The listing builds one solid part. Answer for the finished solid, in the listing's coordinates (mm). A direction names the side the tool comes from. Give positions to 0.01 mm unless a question says otherwise; leave off trailing zeros. Order: outer loops, then holes, each group sorted by start corner. A loop starts at its lowest first (then second) coordinate and runs counter-clockwise, first axis right, second up. Notation, with made-up numbers: (-21, 12.5) - (24, 12.5) arc R28 ccw to (24, 38.5) - close; hole circle Ø1 at (8.5, 36). An arc over 180 degrees is marked (long way). Answer in a Markdown table with one row per item.
from build123d import *

# Parameters (mm, degrees)
SKETCH1_R               = 26.19375
BOSS_EXTRUDE1_DEPTH     = 8.397875
SKETCH2_R               = 12.7
BOSS_EXTRUDE2_DEPTH     = 15.08125
BOSS_EXTRUDE3_START     = 6.35
SKETCH3_R               = 26.19375
BOSS_EXTRUDE3_DEPTH     = 6.35
F_1_4_20_TAPPED_HOLE1_D = 5.1054
SKETCH6_W               = 66.50359939
SKETCH6_H               = 67.616646228
CUT_EXTRUDE2_DEPTH      = 7.9375


with BuildPart() as part:
    # Sketch1 → Boss-Extrude1 (new body)
    with BuildSketch(Plane(origin=(0, 0, 0), x_dir=(1, 0, 0), z_dir=(0, 1, 0))):
        with Locations(Location((0, 0, 0), (0, 0, 270))):
            Circle(SKETCH1_R)
    extrude(amount=-BOSS_EXTRUDE1_DEPTH)

    # Sketch2 → Boss-Extrude2 (add)
    with BuildSketch(Plane.XZ.offset(8.397875)):
        with Locations(Location((0, 0, 0), (0, 0, 90))):
            Circle(SKETCH2_R)
    extrude(amount=BOSS_EXTRUDE2_DEPTH)

    # Sketch3 → Boss-Extrude3 (add)
    with BuildSketch(Plane(origin=(0, 0, 0), x_dir=(1, 0, 0), z_dir=(0, 1, 0)).offset(BOSS_EXTRUDE3_START)):
        with Locations(Location((0, 0, 0), (0, 0, 270))):
            Circle(SKETCH3_R)
        with BuildLine():
            ThreePointArc((2.553003524, 16.40046245), (5.651302793, 17.39292157), (7.574526721, 14.768870658))
            ThreePointArc((7.574526721, 14.768870658), (7.926495509, 13.34211974), (8.883198518, 12.226673836))
            ThreePointArc((8.883198518, 12.226673836), (10.239688102, 11.661486946), (11.705373197, 11.767635017))
            ThreePointArc((11.705373197, 11.767635017), (14.795302793, 10.749416694), (14.808845207, 7.496072251))
            ThreePointArc((14.808845207, 7.496072251), (14.25497079, 6.134924448), (14.373317131, 4.670173836))
            ThreePointArc((14.373317131, 4.670173836), (15.138531738, 3.415603465), (16.386688159, 2.639970974))
            ThreePointArc((16.386688159, 2.639970974), (18.288, 0), (16.386688159, -2.639970974))
            ThreePointArc((16.386688159, -2.639970974), (15.138531738, -3.415603465), (14.373317131, -4.670173836))
            ThreePointArc((14.373317131, -4.670173836), (14.25497079, -6.134924448), (14.808845207, -7.496072251))
            ThreePointArc((14.808845207, -7.496072251), (14.795302793, -10.749416694), (11.705373197, -11.767635017))
            ThreePointArc((11.705373197, -11.767635017), (10.239688102, -11.661486946), (8.883198518, -12.226673836))
            ThreePointArc((8.883198518, -12.226673836), (7.926495509, -13.34211974), (7.574526721, -14.768870658))
            ThreePointArc((7.574526721, -14.768870658), (5.651302793, -17.39292157), (2.553003524, -16.40046245))
            ThreePointArc((2.553003524, -16.40046245), (1.429631644, -15.453078773), (0, -15.113))
            ThreePointArc((0, -15.113), (-1.429631644, -15.453078773), (-2.553003524, -16.40046245))
            ThreePointArc((-2.553003524, -16.40046245), (-5.651302793, -17.39292157), (-7.574526721, -14.768870658))
            ThreePointArc((-7.574526721, -14.768870658), (-7.926495509, -13.34211974), (-8.883198518, -12.226673836))
            ThreePointArc((-8.883198518, -12.226673836), (-10.239688102, -11.661486946), (-11.705373197, -11.767635017))
            ThreePointArc((-11.705373197, -11.767635017), (-14.795302793, -10.749416694), (-14.808845207, -7.496072251))
            ThreePointArc((-14.808845207, -7.496072251), (-14.25497079, -6.134924448), (-14.373317131, -4.670173836))
            ThreePointArc((-14.373317131, -4.670173836), (-15.138531738, -3.415603465), (-16.386688159, -2.639970974))
            ThreePointArc((-16.386688159, -2.639970974), (-18.288, 0), (-16.386688159, 2.639970974))
            ThreePointArc((-16.386688159, 2.639970974), (-15.138531738, 3.415603465), (-14.373317131, 4.670173836))
            ThreePointArc((-14.373317131, 4.670173836), (-14.25497079, 6.134924448), (-14.808845207, 7.496072251))
            ThreePointArc((-14.808845207, 7.496072251), (-14.795302793, 10.749416694), (-11.705373197, 11.767635017))
            ThreePointArc((-11.705373197, 11.767635017), (-10.239688102, 11.661486946), (-8.883198518, 12.226673836))
            ThreePointArc((-8.883198518, 12.226673836), (-7.926495509, 13.34211974), (-7.574526721, 14.768870658))
            ThreePointArc((-7.574526721, 14.768870658), (-5.651302793, 17.39292157), (-2.553003524, 16.40046245))
            ThreePointArc((-2.553003524, 16.40046245), (-1.429631644, 15.453078773), (0, 15.113))
            ThreePointArc((0, 15.113), (1.429631644, 15.453078773), (2.553003524, 16.40046245))
        make_face(mode=Mode.SUBTRACT)
    extrude(amount=-BOSS_EXTRUDE3_DEPTH)

    # 1/4-20 Tapped Hole1 (through all)
    with Locations(Plane(origin=(0, -23.479125, 0), x_dir=(-1, 0, 0), z_dir=(0, -1, 0))):
        with Locations((0, 6.35), (5.499261314, -3.175), (-5.499261314, -3.175)):
            Hole(F_1_4_20_TAPPED_HOLE1_D / 2)

    # Sketch6 → Cut-Extrude2 (cut)
    with BuildSketch(Plane(origin=(0, 6.35, 0), x_dir=(1, 0, 0), z_dir=(0, 1, 0))):
        Rectangle(SKETCH6_W, SKETCH6_H)
        with BuildLine():
            ThreePointArc((26.19375, 0), (2.38125, -23.8125), (-21.43125, 0))
            ThreePointArc((-21.43125, 0), (2.38125, 23.8125), (26.19375, 0))
        make_face(mode=Mode.SUBTRACT)
    extrude(amount=-CUT_EXTRUDE2_DEPTH, mode=Mode.SUBTRACT)


solid = part.part
Item 1: Each of these flat-tipped pins is pushed along its axis until it touches: P1, Ø1.5, axis at x = -5.5, y = -0.5, coming from the -Z side; P2, Ø8, axis at x = 17, z = 2.5, coming from the -Y side; P3, Ø6, axis at x = 4, y = -6.5, coming from the -Z side. Where does it stop, or does it pass through?
Answer block:
| item | result |
|---|---|
| P1 | z = -22.72 |
| P2 | y = -8.4 |
| P3 | z = -26.17 |
Item 2: Consider line 1 (X direction, y = -1, z = 3.5); line 2 (Z direction, x = 0, y = -5.25); line 3 (Z direction, x = -12, y = 5.25). Determine where each line is inside the solid, lowest interval first.
Answer block:
| item | result |
|---|---|
| line 1 | -21.17 to -8.03, -2.97 to 2.97, 8.03 to 25.94 |
| line 2 | -26.19 to -8.9, -3.8 to 26.19 |
| line 3 | -18.98 to -11.84, 11.84 to 18.98 |
Item 3: Find section D-D on y = -12. Write down the section's boundary in (x, z) (3 decimals).
Answer block:
| item | result |
|---|---|
| outline | circle Ø25.4 at (0, 0); hole circle Ø5.105 at (-5.499, 3.175); hole circle Ø5.105 at (0, -6.35); hole circle Ø5.105 at (5.499, 3.175) |
Item 4: Find section C-C on z = -23. Write down the section's boundary in (x, y), then the cut area to 3 significant figures.
Answer block:
| item | result |
|---|---|
| outline | (-12.53, -8.4) - (12.53, -8.4) - (12.53, -1.59) - (8.55, -1.59) - (8.55, 6.35) - (-3.79, 6.35) - (-3.79, -1.59) - (-12.53, -1.59) - close |
| area | 269 mm² |
Item 5: Which of the six approach directions +Z, -Z, +X, -X, +Y, -Y give full straight-line access (tool end or side, diameter ignored) to faces 5 (the face through (7.934, -11.575, 2.408)), 6 (the face through (-5.697, 3.219, -17.377))?
Answer block:
| item | result |
|---|---|
| face 5 | +Y, -Y |
| face 6 | +Y |
Item 6: Find section A-A on z = -6.35. Write down the section's boundary in (x, y).
Answer block:
| item | result |
|---|---|
| outline | (-25.41, -8.4) - (-11, -8.4) - (-11, -23.48) - (-2.55, -23.48) - (-2.55, 0) - (-14.3, 0) - (-14.3, 6.35) - (-20.57, 6.35) - (-20.57, -1.59) - (-25.41, -1.59) - close; (2.55, -23.48) - (11, -23.48) - (11, -8.4) - (25.41, -8.4) - (25.41, -1.59) - (25.33, -1.59) - (25.33, 6.35) - (14.3, 6.35) - (14.3, 0) - (2.55, 0) - close |
Item 7: Determine the mould class of faces 1 (the face through (19, 6.35, 0)), 2 (the face through (0, 0, 0)), 3 (the face through (7.543, 2.437, 23.246)), 4 (the face through (18.288, 3.219, -0.049)) for opening direction X: pulls with the +X half, pulls with the -X half, needs draft (parallel to the pull), parting line crosses it, or undercut.
Answer block:
| item | result |
|---|---|
| face 1 | needs draft |
| face 2 | undercut |
| face 3 | parting line crosses it |
| face 4 | undercut |
